The drawing under review shows one solid part. Ordinate dimensions are in mm from its lowest x, y, z. A direction names the side the tool comes from. Coordinates: 2 decimals unless noted, no trailing zeros. Loops run counter-clockwise (first coordinate to the right, second up) from the corner with the lowest first, then second, coordinate; pieces in that order, holes last.
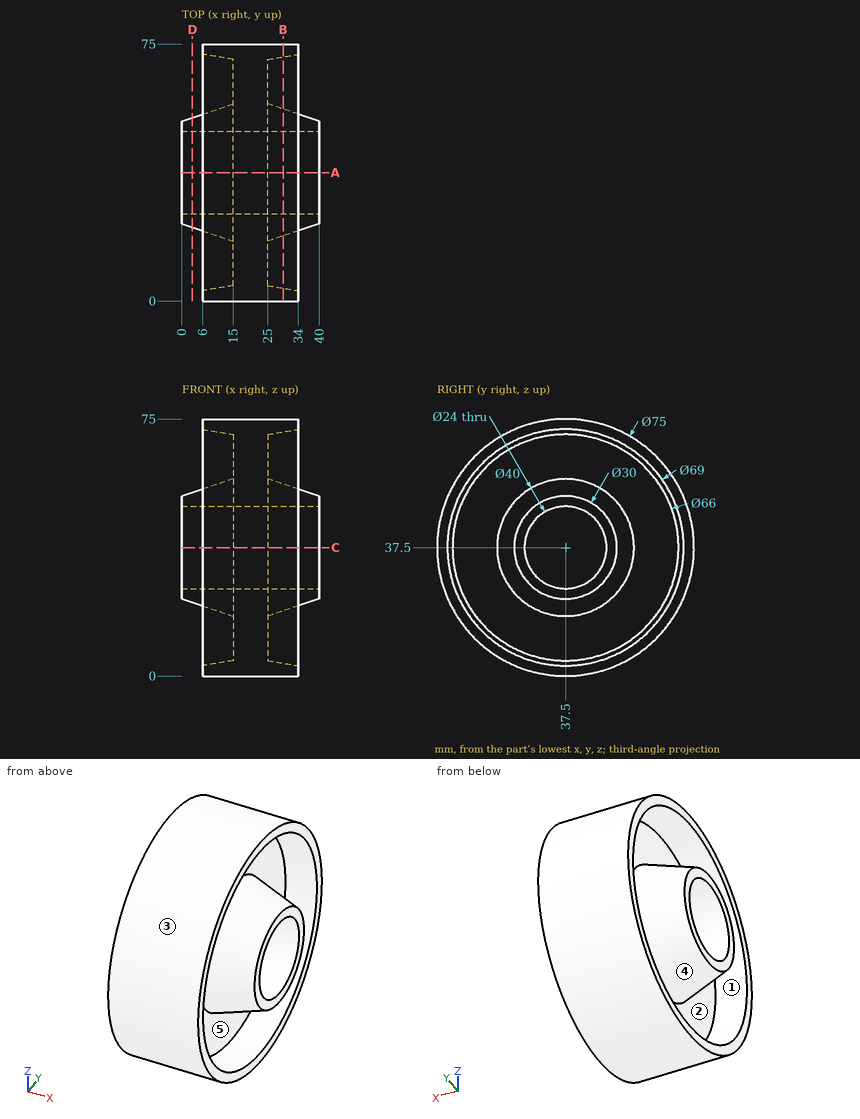
Q1. Take a section at A-A, the plane y = 37.5. Write out the cut boundary in (x, z).
Q2. Take a section at D-D, the plane x = 3. Write out the cut boundary in (y, z), then the cut area to 3 significant figures.
Q3. The part is to be moulded in two halves that separate along Z. For the marked faces 1, 2 and 3, say which applies: pulls with the +Z half, pulls with the -Z half, needs draft (parallel to the pull), parting line crosses it, or undercut.
Q4. Machinability: for the marked faces 4 and 5, which of the approach directions +Z, -Z, +X, -X, +Y, -Y give a long, thin tool a straight path to every point of the face, cutting with its end or side? Answer none if there is none.
Q5. Clearance check with flat-ended pins moving along their axes: pin 1 Ø2 at (x, y) = (10, 48.5) entering from +Z; pin 2 Ø8 at (y, z) = (65, 51.5) entering from -X; pin 3 Ø5 at (y, z) = (25, 57) entering from +X; pin 4 Ø19 at (y, z) = (37.5, 37.5) entering from +X. State where each tip first meets the part, or that it passes through.
Q6. Take a section at B-B, the plane x = 29.5. Write out the cut boundary in (y, z).
Q7. For line 1 (Z direction, x = 9, y = 37); line 2 (Y direction, x = 29, z = 37.5); line 3 (Y direction, x = 28, z = 37), list the stretches that pass through material, from the lowest coordinate up.
Entries:
1. outline: (0, 22.5) - (15, 17.5) - (15, 4.5) - (6, 3) - (6, 0) - (34, 0) - (34, 3) - (25, 4.5) - (25, 17.5) - (40, 22.5) - (40, 25.5) - (0, 25.5) - close; (0, 49.5) - (40, 49.5) - (40, 52.5) - (25, 57.5) - (25, 70.5) - (34, 72) - (34, 75) - (6, 75) - (6, 72) - (15, 70.5) - (15, 57.5) - (0, 52.5) - close
2. outline: circle Ø32 at (37.5, 37.5); hole circle Ø24 at (37.5, 37.5)
2. area: 352 mm2
3. face 1: undercut
3. face 2: undercut
3. face 3: parting line crosses it
4. face 4: -X
4. face 5: +X
5. pin 1: stops at z = 73.64
5. pin 2: stops at x = 6
5. pin 3: stops at x = 25
5. pin 4: passes through
6. outline: circle Ø75 at (37.5, 37.5); circle Ø37 at (37.5, 37.5); hole circle Ø67.5 at (37.5, 37.5); hole circle Ø24 at (37.5, 37.5)
7. line 1: z = 0 to 3.5, 19.51 to 25.51, 49.49 to 55.49, 71.5 to 75
7. line 2: y = 0 to 3.83, 18.83 to 25.5, 49.5 to 56.17, 71.17 to 75
7. line 3: y = 0 to 4, 18.51 to 25.51, 49.49 to 56.49, 71 to 75
